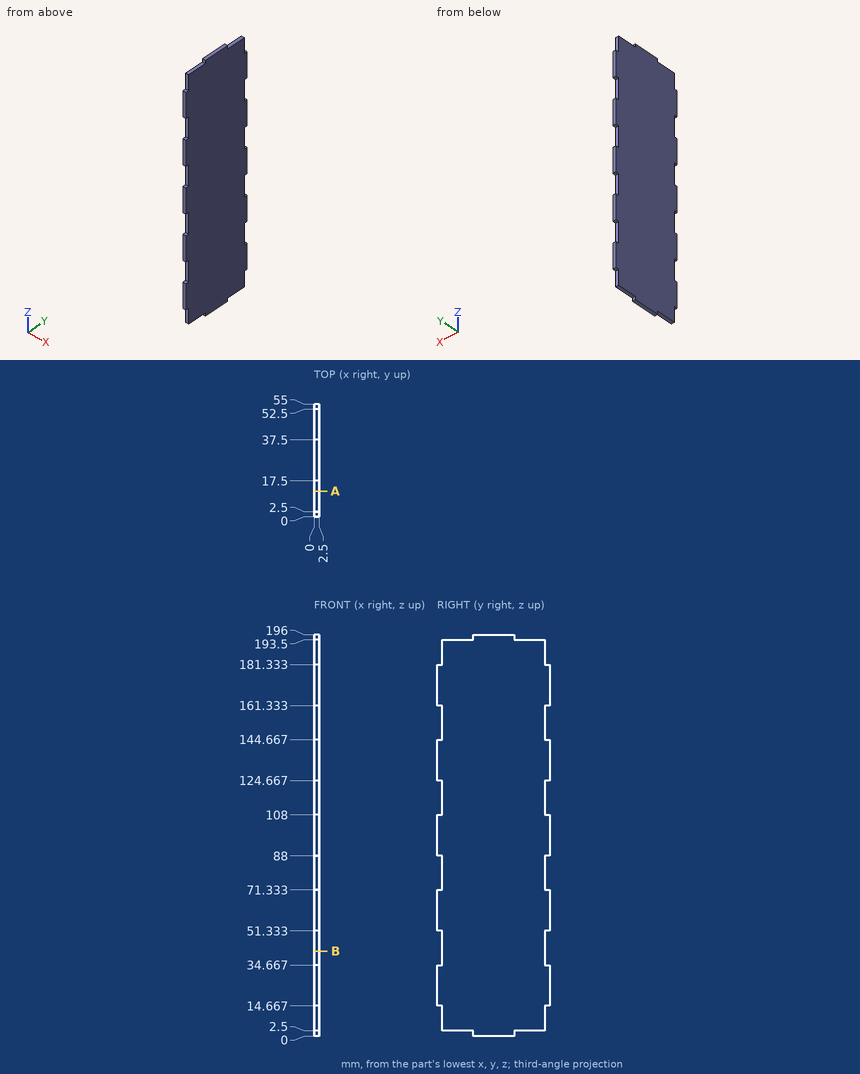
Check sheet for the drawn part. Datum: minimum x, y, z corner. Units: mm. Give positions to 0.01 mm unless a question says otherwise; leave off trailing zeros. Write each loop counter-clockwise with the first axis right and the second up, starting at its lowest first coordinate (ties: lowest second). Pieces come first, ordered by that corner, then holes.
(1) Material ranges on line 1 (Y direction, x = 1.2, z = 36); line 2 (Z direction, x = 1.3, y = 15), recorded low to high.
(2) Cross-section at A-A (y = 12.5). Enter the section's corners in (x, z).
(3) Cross-section at B-B (z = 41.5). Enter the section's corners in (x, y).
(4) Gauge pin test, flat ends, axial feed: pin 1 (0.8 mm diameter, centred on x = 1.5, y = 1.5, fed in from +Z); pin 2 (0.8 mm diameter, centred on x = 1.5, y = 1, fed in from -Z); pin 3 (1 mm diameter, centred on x = 1.5, z = 116.5, fed in from -Y). Record the tip position at first contact, or that the pin passes through.
Worked out:
1. line 1: y = 2.5 to 52.5
1. line 2: z = 2.5 to 193.5
2. outline: (0, 2.5) - (2.5, 2.5) - (2.5, 193.5) - (0, 193.5) - close
3. outline: (0, 2.5) - (2.5, 2.5) - (2.5, 52.5) - (0, 52.5) - close
4. pin 1: stops at z = 181.33
4. pin 2: stops at z = 14.67
4. pin 3: stops at y = 2.5
